from build123d import *

# Parameters (mm, degrees)
CROQUIS1_W              = 45.5
CROQUIS1_H              = 20
SALIENTE_EXTRUIR1_DEPTH = 3.3
CROQUIS2_R              = 7.95
SALIENTE_EXTRUIR2_DEPTH = 11.5
CROQUIS3_R              = 5.95
CORTAR_EXTRUIR1_DEPTH   = 6.5
CROQUIS4_W              = 10
CROQUIS4_H              = 2.5
SALIENTE_EXTRUIR3_DEPTH = 2.5
CROQUIS5_W              = 2.4
CROQUIS5_H              = 2.4
SALIENTE_EXTRUIR4_DEPTH = 2
CROQUIS6_W              = 2.4
CROQUIS6_H              = 1.5
SALIENTE_EXTRUIR5_DEPTH = 5.3


with BuildPart() as part:
    # Croquis1 → Saliente-Extruir1 (new body)
    with BuildSketch(Plane.XY):
        with Locations((22.75, 10)):
            Rectangle(CROQUIS1_W, CROQUIS1_H)
    extrude(amount=SALIENTE_EXTRUIR1_DEPTH)

    # Croquis2 → Saliente-Extruir2 (add)
    with BuildSketch(Plane.XY.offset(3.3)):
        with Locations((34.125, 10)):
            Circle(CROQUIS2_R)
        with Locations((11.375, 10)):
            Circle(CROQUIS2_R)
    extrude(amount=SALIENTE_EXTRUIR2_DEPTH)

    # Croquis3 → Cortar-Extruir1 (cut)
    with BuildSketch(Plane.XY.offset(14.8)):
        with Locations((34.125, 10)):
            Circle(CROQUIS3_R)
        with Locations((11.375, 10)):
            Circle(CROQUIS3_R)
    extrude(amount=-CORTAR_EXTRUIR1_DEPTH, mode=Mode.SUBTRACT)

    # Croquis4 → Saliente-Extruir3 (add)
    with BuildSketch(Plane(origin=(0, 0, 0), x_dir=(-1, 0, 0), z_dir=(0, 0, -1))):
        with Locations((-22.5, 1.25)):
            Rectangle(CROQUIS4_W, CROQUIS4_H)
    extrude(amount=SALIENTE_EXTRUIR3_DEPTH)

    # Croquis5 → Saliente-Extruir4 (add)
    with BuildSketch(Plane(origin=(0, 0, -2.5), x_dir=(-1, 0, 0), z_dir=(0, 0, -1))):
        with Locations((-26.235, 1.25)):
            Rectangle(CROQUIS5_W, CROQUIS5_H)
        with Locations((-23.745, 1.25)):
            Rectangle(CROQUIS5_W, CROQUIS5_H)
        with Locations((-21.255, 1.25)):
            Rectangle(CROQUIS5_W, CROQUIS5_H)
        with Locations((-18.765, 1.25)):
            Rectangle(CROQUIS5_W, CROQUIS5_H)
    extrude(amount=SALIENTE_EXTRUIR4_DEPTH)

    # Croquis6 → Saliente-Extruir5 (add)
    with BuildSketch(Plane.XZ.offset(-0.05)):
        with Locations((18.765, -3.75)):
            Rectangle(CROQUIS6_W, CROQUIS6_H)
        with Locations((21.255, -3.75)):
            Rectangle(CROQUIS6_W, CROQUIS6_H)
        with Locations((23.745, -3.75)):
            Rectangle(CROQUIS6_W, CROQUIS6_H)
        with Locations((26.235, -3.75)):
            Rectangle(CROQUIS6_W, CROQUIS6_H)
    extrude(amount=SALIENTE_EXTRUIR5_DEPTH)


solid = part.part
Geometry check sheet. Reference: the model listing, model coordinates, mm. A direction names the side the tool comes from. Round coordinates to 2 decimals unless told otherwise and drop trailing zeros. Write each loop counter-clockwise with the first axis right and the second up, starting at its lowest first coordinate (ties: lowest second). Pieces come first, ordered by that corner, then holes. Notation, with made-up numbers: (42, 59) - (47, 59) arc R19 ccw to (47, 87) - close; hole circle Ø5 at (87, 81.5). An arc over 180 degrees is marked (long way). One line per item, written item: value.
1. Depth check by flat-ended pin: pin 1 Ø1.5 at (x, y) = (27.5, 7) entering from -Z; pin 2 Ø0.6 at (x, z) = (21, -2.5) entering from -Y; pin 3 Ø2.5 at (x, y) = (19.5, -2) entering from +Z; pin 4 Ø1.5 at (y, z) = (17, -1) entering from +X. Enter the tip coordinate at first touch or a pass-through.
The answers:
pin 1: stops at z = 0
pin 2: stops at y = 0
pin 3: stops at z = -3
pin 4: passes through
2. Set-up check for faces 1 (the face through (27.435, -1, -4)), 2 (the face through (22, 0, 1)), 3 (the face through (24, 2.45, -3)), 4 (the face through (11, 10, 8.3)): record each of +Z, -Z, +X, -X, +Y, -Y from which the full face is reachable in a straight line by a thin tool's end or side.
The answers:
face 1: -Z, +X, +Y, -Y
face 2: +Z, +X, -X, -Y
face 3: -Z, +X, -X, +Y
face 4: +Z
3. Cross-section at D-D on z = 6.5. Record the boundary of the cut face in (x, y) (3 decimals), and give its area (3 significant figures).
The answers:
outline: circle Ø15.9 at (11.375, 10); circle Ø15.9 at (34.125, 10)
area: 397 mm^2
4. Cross-section at B-B on z = 10.75. Record the boundary of the cut face in (x, y) (3 decimals).
The answers:
outline: circle Ø15.9 at (11.375, 10); circle Ø15.9 at (34.125, 10); hole circle Ø11.9 at (11.375, 10); hole circle Ø11.9 at (34.125, 10)
5. Scan lines: L1, parallel to X at y = 15.5, z = 9.5; L2, parallel to X at y = 11.5, z = 8.5; L3, parallel to Z at x = 30.5, y = 8.5. Record each from-to range of solid material in increasing order.
The answers:
L1: x = 5.63 to 9.11, 13.64 to 17.12, 28.38 to 31.86, 36.39 to 39.87
L2: x = 3.57 to 5.62, 17.13 to 19.18, 26.32 to 28.37, 39.88 to 41.93
L3: z = 0 to 8.3
6. Cross-section at C-C on y = 10. Record the boundary of the cut face in (x, z) (3 decimals), and give its area (3 significant figures).
The answers:
outline: (0, 0) - (45.5, 0) - (45.5, 3.3) - (42.075, 3.3) - (42.075, 14.8) - (40.075, 14.8) - (40.075, 8.3) - (28.175, 8.3) - (28.175, 14.8) - (26.175, 14.8) - (26.175, 3.3) - (19.325, 3.3) - (19.325, 14.8) - (17.325, 14.8) - (17.325, 8.3) - (5.425, 8.3) - (5.425, 14.8) - (3.425, 14.8) - (3.425, 3.3) - (0, 3.3) - close
area: 361 mm^2
7. Cross-section at A-A on x = 21.5. Record the boundary of the cut face in (y, z).
The answers:
outline: (-5.25, -4.5) - (2.45, -4.5) - (2.45, -2.5) - (2.5, -2.5) - (2.5, 0) - (20, 0) - (20, 3.3) - (0, 3.3) - (0, -2.5) - (0.05, -2.5) - (0.05, -3) - (-5.25, -3) - close
